from build123d import *

# Parameters (mm, degrees)
EXTRUDE_1_DEPTH = 60
SKETCH_2_R      = 2
EXTRUDE_2_DEPTH = 6
M4X0_7_1_D      = 3.3
M4X0_7_1_DEPTH  = 10.5
M4X0_7_1_TIP    = 0.991420021


with BuildPart() as part:
    # 草圖1 → 填料-伸長1 (new body)
    with BuildSketch(Plane.XY):
        Polygon((4.041451884, 0), (2.020725942, 3.5), (-2.020725942, 3.5), (-4.041451884, 0), (-2.020725942, -3.5), (2.020725942, -3.5), align=None)
    extrude(amount=EXTRUDE_1_DEPTH)

    # 草圖2 → 填料-伸長2 (add)
    with BuildSketch(Plane.XY.offset(60)):
        Circle(SKETCH_2_R)
    extrude(amount=EXTRUDE_2_DEPTH)

    # M4x0.7 螺紋孔1
    with Locations(Plane(origin=(0, 0, 0), x_dir=(-1, 0, 0), z_dir=(0, 0, -1))):
        with Locations((0, 0)):
            Hole(M4X0_7_1_D / 2, depth=M4X0_7_1_DEPTH)
            with Locations((0, 0, -(M4X0_7_1_DEPTH + M4X0_7_1_TIP / 2))):  # 118° drill point
                Cone(0, M4X0_7_1_D / 2, M4X0_7_1_TIP, mode=Mode.SUBTRACT)


solid = part.part
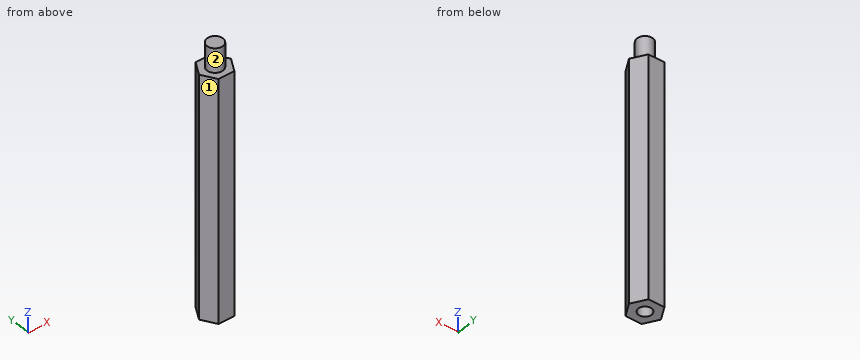
Design review of the part built by this model. Coordinates are the model's own, in mm. Face numbers are marked on the shaded views. A direction names the side the tool comes from. Round coordinates to 2 decimals unless told otherwise and drop trailing zeros. Loops run counter-clockwise (first coordinate to the right, second up) from the corner with the lowest first, then second, coordinate; pieces in that order, holes last. Notation, with made-up numbers: (-29.5, -25.75) - (-24.5, -25.75) arc R22 cw to (-24.5, -19.75) - close; hole circle Ø5 at (31, -26.5). An arc over 180 degrees is marked (long way). One line per question, with ' | ' between items.
1. Clearance check with flat-ended pins moving along their axes: P1, Ø1.5, axis at x = 1.5, y = -2.5, coming from the +Z side; P2, Ø3, axis at x = 0, y = 0, coming from the -Z side. State where each tip first meets the part, or that it passes through.
Results are:
P1: stops at z = 60 | P2: stops at z = 10.59
2. We need section A-A, the plane z = 5.5. State the section outline as (x, y) points.
Results are:
outline: (-4.04, 0) - (-2.02, -3.5) - (2.02, -3.5) - (4.04, 0) - (2.02, 3.5) - (-2.02, 3.5) - close; hole circle Ø3.3 at (0, 0)
3. For the marked faces 1 and 2, list the 3-axis set-ups (+Z, -Z, +X, -X, +Y, -Y) from which the entire face can be reached by the end or side of a thin tool; tool diameter is ignored.
Results are:
face 1: +Z, -Z, -X, -Y | face 2: +Z
4. We need section D-D, the plane y = 2.75. State the section outline as (x, z) points.
Results are:
outline: (-2.45, 0) - (2.45, 0) - (2.45, 60) - (-2.45, 60) - close
5. We need section B-B, the plane z = 49.5. State the section outline as (x, y) points.
Results are:
outline: (-4.04, 0) - (-2.02, -3.5) - (2.02, -3.5) - (4.04, 0) - (2.02, 3.5) - (-2.02, 3.5) - close
6. We need section C-C, the plane x = 3. State the section outline as (y, z) points.
Results are:
outline: (-1.8, 0) - (1.8, 0) - (1.8, 60) - (-1.8, 60) - close
7. For L1, parallel to X at y = 0, z = 5; L2, parallel to Y at x = 0, z = 5; L3, parallel to Z at x = -1.5, y = 3.25, list the stretches that pass through material, from the lowest coordinate up. Write a range as [from, to].
Results are:
L1: x = [-4.04, -1.65], [1.65, 4.04] | L2: y = [-3.5, -1.65], [1.65, 3.5] | L3: z = [0, 60]
